```python
from build123d import *

# Parameters (mm, degrees)
BOSS_EXTRUDE1_DEPTH = 8.89
SKETCH5_R           = 19.05
CUT_EXTRUDE2_DEPTH  = 22.59


with BuildPart() as part:
    # Sketch1 → Boss-Extrude1 (new body)
    with BuildSketch(Plane(origin=(0, 0, 0), x_dir=(1, 0, 0), z_dir=(0, 1, 0))):
        with BuildLine():
            Line((44.45, -50.8), (-44.45, -50.8))
            ThreePointArc((-44.45, -50.8), (-48.940128061, -48.940128061), (-50.8, -44.45))
            Line((-50.8, -44.45), (-50.8, 44.45))
            ThreePointArc((-50.8, 44.45), (-48.940128061, 48.940128061), (-44.45, 50.8))
            Line((-44.45, 50.8), (44.45, 50.8))
            ThreePointArc((44.45, 50.8), (48.940128061, 48.940128061), (50.8, 44.45))
            Line((50.8, 44.45), (50.8, -44.45))
            ThreePointArc((50.8, -44.45), (48.940128061, -48.940128061), (44.45, -50.8))
        make_face()
    extrude(amount=BOSS_EXTRUDE1_DEPTH)

    # Sketch2 → Revolve1 (revolve)
    with BuildSketch(Plane.XY):
        Polygon((0, 8.89), (0, 21.59), (25.4, 21.59), (41.275, 8.89), align=None)
    revolve(axis=Axis((0, 37.971899969, 0), (0, -1, 0)))

    # Sketch5 → Cut-Extrude2 (cut, through all)
    with BuildSketch(Plane(origin=(0, 21.59, 0), x_dir=(1, 0, 0), z_dir=(0, 1, 0))):
        with Locations((0, 50.8)):
            Circle(SKETCH5_R)
        with Locations((50.8, 0)):
            Circle(SKETCH5_R)
        with Locations((0, -50.8)):
            Circle(SKETCH5_R)
        with Locations((-50.8, 0)):
            Circle(SKETCH5_R)
    extrude(amount=-CUT_EXTRUDE2_DEPTH, mode=Mode.SUBTRACT)

    # Sketch6 → Revolve2 (revolve)
    with BuildSketch(Plane.XY):
        Polygon((0, 21.59), (25.4, 21.59), (12.7, 339.09), (0, 339.09), align=None)
    revolve(axis=Axis((0, 0, 0), (0, 1, 0)))


solid = part.part
```
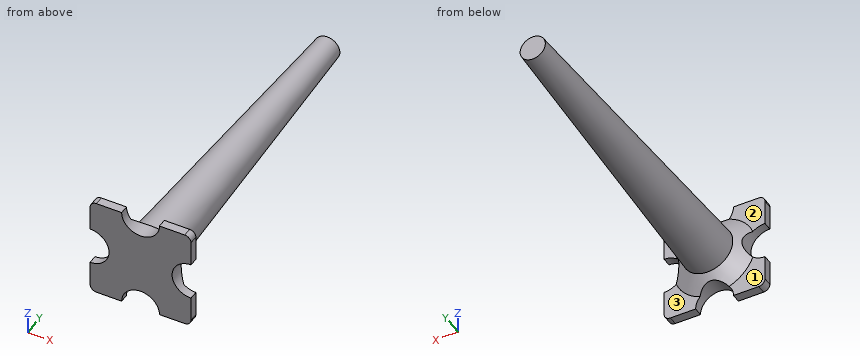
Geometry check sheet. Reference: the model listing, model coordinates, mm. Face numbers are marked on the shaded views. A direction names the side the tool comes from. Coordinates: 2 decimals unless noted, no trailing zeros. Loops run counter-clockwise (first coordinate to the right, second up) from the corner with the lowest first, then second, coordinate; pieces in that order, holes last.
Item 1: Sectioned sample at B-B, the plane x = 0. Record the boundary of the cut face in (y, z).
Item 2: Go/stop test with flat-tipped pins: pin 1 Ø11 at (x, z) = (26, 33) entering from +Y; pin 2 Ø12 at (y, z) = (107.5, -26) entering from +X; pin 3 Ø10 at (y, z) = (250, -9) entering from +X; pin 4 Ø2 at (x, z) = (-21, -16) entering from -Y. Record where each tip stops, or that it passes through.
Item 3: Thickness scan on line 1 (Y direction, x = -32.5, z = 38); line 2 (Z direction, x = -3.5, y = 62.5); line 3 (X direction, y = 42.5, z = -12). Record the ranges inside material, lowest first.
Item 4: Sectioned sample at A-A, the plane z = 0. Record the boundary of the cut face in (x, y).
Item 5: Access from +Z, -Z, +X, -X, +Y, -Y to the whole of each face (thin tool, end or side, straight path). Record for the marked faces 1, 2 and 3.
Item 6: Sectioned sample at D-D, the plane y = 55.5. Record the boundary of the cut face in (x, z).
Item 7: Sectioned sample at C-C, the plane y = 169.5. Record the boundary of the cut face in (x, z).
Check result:
1. outline: (0, -31.75) - (16.51, -31.75) - (21.59, -25.4) - (339.09, -12.7) - (339.09, 12.7) - (21.59, 25.4) - (16.51, 31.75) - (0, 31.75) - close
2. pin 1: stops at y = 12.7
2. pin 2: stops at x = 9.09
2. pin 3: stops at x = 15.78
2. pin 4: stops at y = 0
3. line 1: y = 0 to 8.89
3. line 2: z = -23.5 to 23.5
3. line 3: x = -21.43 to 21.43
4. outline: (-31.75, 0) - (31.75, 0) - (31.75, 16.51) - (25.4, 21.59) - (12.7, 339.09) - (-12.7, 339.09) - (-25.4, 21.59) - (-31.75, 16.51) - close
5. face 1: -Z, -X, +Y
5. face 2: +Z, -X, +Y
5. face 3: -Z, +X, +Y
6. outline: circle Ø48.09 at (0, 0)
7. outline: circle Ø38.97 at (0, 0)
